from build123d import *

# Parameters (mm, degrees)
F0_R       = 2.1666665
F1_DEPTH   = 5.5
F2_SIZE    = 0.75
F3_W       = 51
F3_H       = 8
F4_DEPTH   = 5.5
F5_SIZE    = 0.5
F7_R       = 5
F8_SIZE2   = 2
F8_SIZE    = 3
F8_2_SIZE2 = 2
F8_2_SIZE  = 3


with BuildPart() as f1:
    # F0 (on Top) → F1 (new body)
    with BuildSketch(Plane.XY):
        with BuildLine():
            Line((25.5, 11), (-25.5, 11))
            Line((-25.5, 11), (-25.5, -11))
            Line((-25.5, -11), (-10.625, -11))
            Line((-10.625, -11), (-10.625, -0.2))
            ThreePointArc((-10.625, -0.2), (-4.425, 6), (1.775, -0.2))
            Line((1.775, -0.2), (1.775, -11))
            Line((1.775, -11), (25.5, -11))
            Line((25.5, -11), (25.5, 11))
        make_face()
        with Locations((-20.75, 0)):
            Circle(F0_R, mode=Mode.SUBTRACT)
        with Locations((21, 0)):
            Circle(F0_R, mode=Mode.SUBTRACT)
    extrude(amount=F1_DEPTH)

    # F2
    f2_edges = [f1.edges().sort_by_distance(p)[0] for p in [
        (-22.916666, 0, 0),
        (18.833334, 0, 0),
        (18.833334, 0, 5.5),
        (-22.916666, 0, 5.5),
    ]]
    chamfer(f2_edges, length=F2_SIZE)

    # F3 (on Top) → F4 (join, through all)
    with BuildSketch(Plane.XY):
        with Locations((0, 15)):
            Rectangle(F3_W, F3_H)
    extrude(amount=F4_DEPTH)

    # F5
    f5_edges = [f1.edges().sort_by_distance(p)[0] for p in [
        (-4.425, 6, 5.5),
        (-4.425, 6, 0),
        (-10.625, -5.6, 5.5),
        (-10.625, -5.6, 0),
        (1.775, -5.6, 0),
        (1.775, -5.6, 5.5),
    ]]
    chamfer(f5_edges, length=F5_SIZE)

    # F7
    f7_edges = [f1.edges().sort_by_distance(p)[0] for p in [
        (25.5, -11, 2.75),
        (-25.5, -11, 2.75),
        (25.5, 19, 2.75),
        (-25.5, 19, 2.75),
    ]]
    fillet(f7_edges, radius=F7_R)

    # F8
    f8_edges = [f1.edges().sort_by_distance(p)[0] for p in [
        (-10.625, -11, 2.75),
    ]]
    f8_side = f1.faces().sort_by_distance((-10.625, -5.6, 2.75))[0]
    chamfer(f8_edges, length=F8_SIZE, length2=F8_SIZE2, reference=f8_side)

    # F8#2
    f8_2_edges = [f1.edges().sort_by_distance(p)[0] for p in [
        (1.775, -11, 2.75),
    ]]
    f8_2_side = f1.faces().sort_by_distance((11.159877, -11, 2.75))[0]
    chamfer(f8_2_edges, length=F8_2_SIZE, length2=F8_2_SIZE2, reference=f8_2_side)


solid = f1.part
Can you work these out from the model? Positions are in its coordinate system, mm. A direction names the side the tool comes from. Coordinates: 2 decimals unless noted, no trailing zeros. Write each loop counter-clockwise with the first axis right and the second up, starting at its lowest first coordinate (ties: lowest second). Pieces come first, ordered by that corner, then holes. Notation, with made-up numbers: (87, 12.25) -> (130, 12.25) arc R26 cw to (130, 48.25) -> close; hole circle Ø1 at (85.5, -1.75). An arc over 180 degrees is marked (long way). Write each question's results on one line, items separated by ' | '. Start each with the question number.
Q1. If I drill on probe 1 along Y at (x, z) = (-20.75, 3.5); probe 2 along X at (y, z) = (14.25, 3.95); probe 3 along Y at (x, z) = (22, 0.45), over which ranges is the centre line in solid material (lowest first)?
Q2. I'm going to push a flat-ended pin straight in: pin 1 (2 mm diameter, centred on x = -6, z = 0.5, fed in from -Y). Where does the tip first touch, or does it pass through?
Q3. We'd pull the mould along Y, two halves only. Please class faces 3 (the face through (-4.56, 6, 2.72)), 4 (the face through (-22.915, 0.095, 2.722)), 5 (the face through (-24.07, 17.5, 2.79)), 6 (the face through (-10.625, -4, 3)): +Y half, -Y half, draft (parallel to the pull), parting line (faces both ways), or undercut.
Q4. Imagine slicing it at A-A (z = 3.8). Write out the boundary of the cut face in (x, y) (3 decimals), then the cut area to 3 significant figures.
Q5. Imagine slicing it at B-B (x = 21). Write out the boundary of the cut face in (y, z), then the cut area to 3 significant figures.
Q6. On a 3-axis mill with a long thin cutter (end or side, diameter ignored), from which of +Z, -Z, +X, -X, +Y, -Y can I reach the whole of each face in a straight line? I mean faces 1 (the face through (0, 8, 5.5)), 2 (the face through (1.775, -5, 3)). Say none if no direction works.
Taken from the geometry:
1) probe 1: y = -10.99 to -2.17, 2.17 to 18.99 | probe 2: x = -25.49 to 25.49 | probe 3: y = -10.77 to -2.25, 2.25 to 18.77
2) pin 1: stops at y = 5.44
3) face 3: -Y half | face 4: undercut | face 5: +Y half | face 6: draft
4) outline: (-25.5, -6) arc R5 ccw to (-20.5, -11) -> (-12.625, -11) -> (-10.625, -8) -> (-10.625, -0.2) arc R6.2 cw to (1.775, -0.2) -> (1.775, -9) -> (4.775, -11) -> (20.5, -11) arc R5 ccw to (25.5, -6) -> (25.5, 14) arc R5 ccw to (20.5, 19) -> (-20.5, 19) arc R5 ccw to (-25.5, 14) -> close; hole circle Ø4.333 at (-20.75, 0); hole circle Ø4.333 at (21, 0) | area: 1,280 mm^2
5) outline: (-10.97, 0) -> (-2.92, 0) -> (-2.17, 0.75) -> (-2.17, 4.75) -> (-2.92, 5.5) -> (-10.97, 5.5) -> close; (2.17, 0.75) -> (2.92, 0) -> (18.97, 0) -> (18.97, 5.5) -> (2.92, 5.5) -> (2.17, 4.75) -> close | area: 140 mm^2
6) face 1: +Z, +X, -X, +Y, -Y | face 2: +Z, -Z, -Y
